Read the model definition and answer for the solid it produces. Units are mm, in the model's axes. Face numbers are marked on the shaded views. A direction names the side the tool comes from. Coordinates: 2 decimals unless noted, no trailing zeros. Loops run counter-clockwise (first coordinate to the right, second up) from the corner with the lowest first, then second, coordinate; pieces in that order, holes last.
from build123d import *

# Parameters (mm, degrees)
F0_W     = 6
F0_H     = 0.3
F1_DEPTH = 3


with BuildPart() as f1:
    # F0 (on Top) → F1 (new body)
    with BuildSketch(Plane.XY):
        with BuildLine():
            Line((28.210546, 3.5), (8.291562, 3.5))
            ThreePointArc((8.291562, 3.5), (-9, 0), (8.291562, -3.5))
            Line((8.291562, -3.5), (28.210546, -3.5))
            ThreePointArc((28.210546, -3.5), (45.502108, 0), (28.210546, 3.5))
        make_face()
        with Locations((0, -3.15)):
            Rectangle(F0_W, F0_H, mode=Mode.SUBTRACT)
        with Locations((36.502108, -3.15)):
            Rectangle(F0_W, F0_H, mode=Mode.SUBTRACT)
        with Locations((0, 3.15)):
            Rectangle(F0_W, F0_H, mode=Mode.SUBTRACT)
        with Locations((36.502108, 3.15)):
            Rectangle(F0_W, F0_H, mode=Mode.SUBTRACT)
    extrude(amount=F1_DEPTH)


solid = f1.part
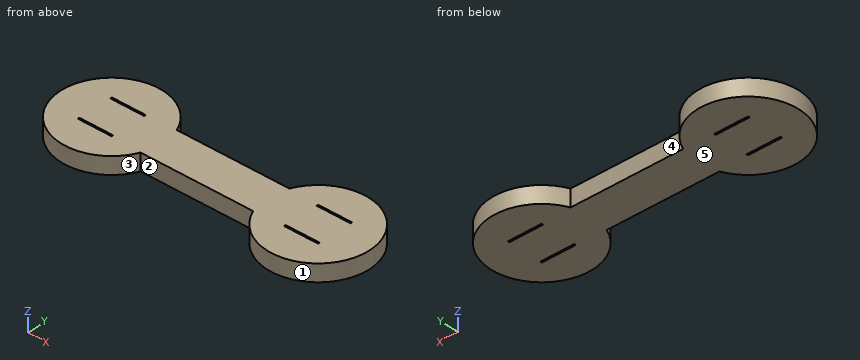
Item 1: Determine the mould class of the marked faces 3, 4 and 5 for opening direction X: released by +X, released by -X, zero draft, split by the parting line, or undercut.
Numbers:
face 3: undercut
face 4: undercut
face 5: zero draft
Item 2: Find the intervals of material crossed by line 1 along Y through (x, z) = (0, 1.15); line 2 along Y through (x, z) = (38.5, 0.85); line 3 along Y through (x, z) = (17.5, 1.1), in increasing order.
Numbers:
line 1: y = -9 to -3.3, -3 to 3, 3.3 to 9
line 2: y = -8.78 to -3.3, -3 to 3, 3.3 to 8.78
line 3: y = -3.5 to 3.5
Item 3: Given pin 1 (0.9 mm diameter, centred on x = 1.5, z = 2, fed in from -Y); pin 2 (1 mm diameter, centred on y = 5, z = 2.5, fed in from +X); pin 3 (1 mm diameter, centred on x = 10, z = 2, fed in from +Y), each flat-ended and moving along its own axis, determine where each tip first touches the part or whether it passes through.
Numbers:
pin 1: stops at y = -8.94
pin 2: stops at x = 44.3
pin 3: stops at y = 3.5
Item 4: A cutting plane is placed at B-B on y = 5.25. Determine the outline of the cut face in (x, z).
Numbers:
outline: (-7.31, 0) - (7.31, 0) - (7.31, 3) - (-7.31, 3) - close; (29.19, 0) - (43.81, 0) - (43.81, 3) - (29.19, 3) - close
Item 5: Which of the six approach directions +Z, -Z, +X, -X, +Y, -Y give full straight-line access (tool end or side, diameter ignored) to the marked faces 1 and 2?
Numbers:
face 1: +Z, -Z
face 2: +Z, -Z, -Y
Item 6: A cutting plane is placed at A-A on x = 0. Determine the outline of the cut face in (y, z), then the cut area to 3 significant figures.
Numbers:
outline: (-9, 0) - (-3.3, 0) - (-3.3, 3) - (-9, 3) - close; (-3, 0) - (3, 0) - (3, 3) - (-3, 3) - close; (3.3, 0) - (9, 0) - (9, 3) - (3.3, 3) - close
area: 52.2 mm2
Item 7: A cutting plane is placed at D-D on y = 8.25. Determine the outline of the cut face in (x, z).
Numbers:
outline: (-3.6, 0) - (3.6, 0) - (3.6, 3) - (-3.6, 3) - close; (32.91, 0) - (40.1, 0) - (40.1, 3) - (32.91, 3) - close
Item 8: A cutting plane is placed at C-C on z = 2.4. Determine the outline of the cut face in (x, y), then the cut area to 3 significant figures.
Numbers:
outline: (8.29, -3.5) - (28.21, -3.5) arc R9 ccw (long way) to (28.21, 3.5) - (8.29, 3.5) arc R9 ccw (long way) to start; hole (-3, -3.3) - (3, -3.3) - (3, -3) - (-3, -3) - close; hole (-3, 3) - (3, 3) - (3, 3.3) - (-3, 3.3) - close; hole (33.5, -3.3) - (39.5, -3.3) - (39.5, -3) - (33.5, -3) - close; hole (33.5, 3) - (39.5, 3) - (39.5, 3.3) - (33.5, 3.3) - close
area: 635 mm2
